```python
from build123d import *

# Parameters (mm, degrees)
F0_R     = 31.5
F0_R_2   = 2.25
F0_R_3   = 11.5
F0_R_4   = 9
F1_DEPTH = 2


with BuildPart() as f1:
    # F0 (on Top) → F1 (new body)
    with BuildSketch(Plane.XY):
        with Locations((0, -7)):
            Circle(F0_R)
        with Locations((-18, -25)):
            Circle(F0_R_2, mode=Mode.SUBTRACT)
        with Locations((18, -25)):
            Circle(F0_R_2, mode=Mode.SUBTRACT)
        with Locations((-18, 11)):
            Circle(F0_R_2, mode=Mode.SUBTRACT)
        with Locations((0, 3)):
            Circle(F0_R_3, mode=Mode.SUBTRACT)
        with Locations((18, 11)):
            Circle(F0_R_2, mode=Mode.SUBTRACT)
        with Locations((0, 3)):
            Circle(F0_R_3)
        with Locations((0, 3)):
            Circle(F0_R_4, mode=Mode.SUBTRACT)
    extrude(amount=-F1_DEPTH)


solid = f1.part
```
Here's how the part is built. I have some questions about the finished solid (model axes, mm). Give positions to 0.01 mm unless a question says otherwise; leave off trailing zeros. Loops run counter-clockwise (first coordinate to the right, second up) from the corner with the lowest first, then second, coordinate; pieces in that order, holes last. Notation, with made-up numbers: M 17.25,57 L 49.25,57 A14 cw 49.25,66 Z; hole C 86,77 d3. An arc over 180 degrees is marked long. Put each result on its own line as item: value. Start each with the question number.
(1) If we mould it in two halves opening along X, with no side actions, what happens to faces 1 (the cylindrical face through (-16.79, 12.897, -0.986)), 2 (the flat face through (0, -7, 0)), 3 (the cylindrical face through (-4.101, 24.232, -0.986)), 4 (the cylindrical face through (-16.962, -26.996, -0.986))? For each: +X half, -X half, draft (parallel to the pull), parting line (faces both ways), or undercut.
(2) I want a section at A-A on x = 0. Please give me the cut outline in (y, z), then the cut area to 3 significant figures.
(3) I want a section at B-B on y = -25. Please give me the cut outline in (x, z).
(4) I need wall thicknesses on line 1 along X through (y, z) = (9, -1.7); line 2 along X through (y, z) = (-25.5, -1.15); line 3 along X through (y, z) = (-27, -0.55). Which ranges of each line are inside material? Lowest first, please. Write a range as [from, to].
(5) I want a section at D-D on y = 3. Please give me the cut outline in (x, z), then the cut area to 3 significant figures.
(6) I want a section at C-C on z = -0.9. Please give me the cut outline in (x, y).
Answer block:
1. face 1: undercut
1. face 2: draft
1. face 3: parting line
1. face 4: undercut
2. outline: M -38.5,-2 L -6,-2 L -6,0 L -38.5,0 Z; M 12,-2 L 24.5,-2 L 24.5,0 L 12,0 Z
2. area: 90.0 mm^2
3. outline: M -25.85,-2 L -20.25,-2 L -20.25,0 L -25.85,0 Z; M -15.75,-2 L 15.75,-2 L 15.75,0 L -15.75,0 Z; M 20.25,-2 L 25.85,-2 L 25.85,0 L 20.25,0 Z
4. line 1: [-27.13, -19.03], [-16.97, -6.71], [6.71, 16.97], [19.03, 27.13]
4. line 2: [-25.5, -20.19], [-15.81, 15.81], [20.19, 25.5]
4. line 3: [-24.34, -19.03], [-16.97, 16.97], [19.03, 24.34]
5. outline: M -29.87,-2 L -9,-2 L -9,0 L -29.87,0 Z; M 9,-2 L 29.87,-2 L 29.87,0 L 9,0 Z
5. area: 83.5 mm^2
6. outline: C 0,-7 d63; hole C -18,-25 d4.5; hole C -18,11 d4.5; hole C 0,3 d18; hole C 18,-25 d4.5; hole C 18,11 d4.5
